Here's the drawing with two shaded views (mm, measured from the low corner). I have some questions. A direction names the side the tool comes from. Coordinates: 2 decimals unless noted, no trailing zeros. Loops run counter-clockwise (first coordinate to the right, second up) from the corner with the lowest first, then second, coordinate; pieces in that order, holes last.
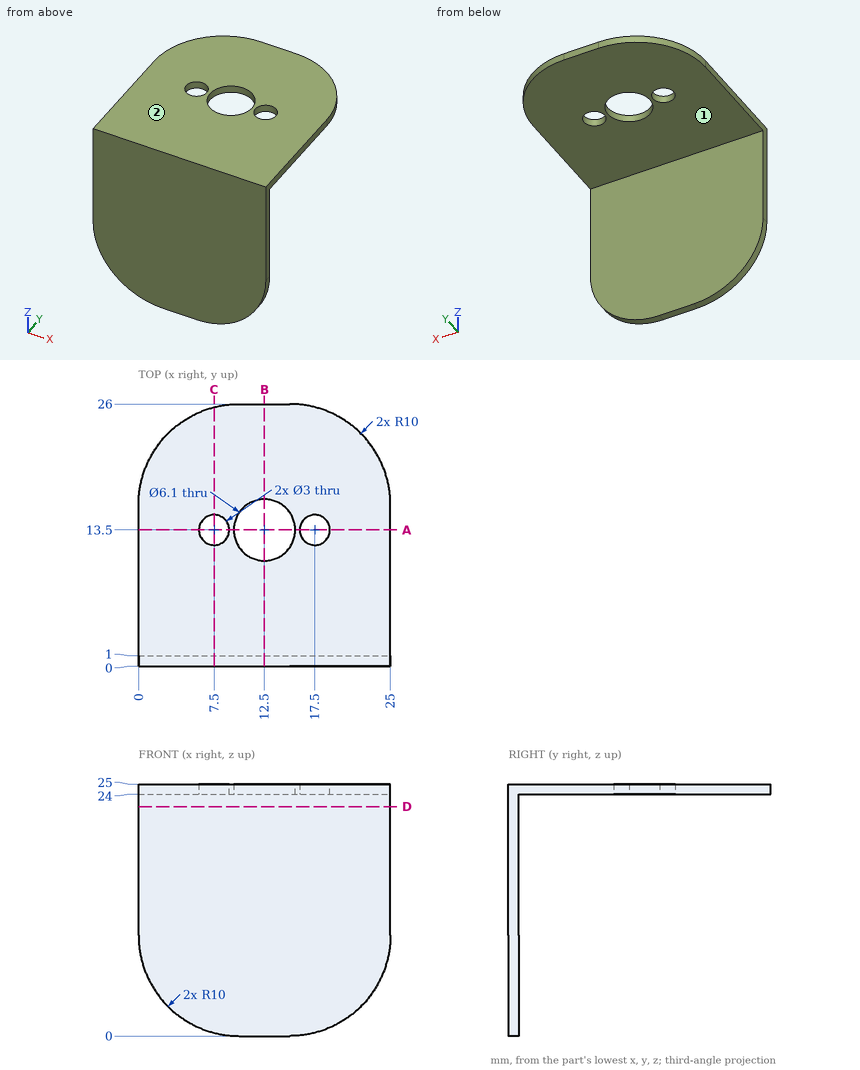
(1) I'm going to push flat-ended pins straight in: pin 1 (2.5 mm diameter, centred on x = 7.5, y = 13.5, fed in from -Z); pin 2 (5 mm diameter, centred on x = 17.5, y = 13.5, fed in from -Z). Where does each tip first touch, or does it pass through?
Check values:
pin 1: passes through
pin 2: stops at z = 24
(2) I want a section at C-C on x = 7.5. Write out the boundary of the cut face in (y, z), then the cut area to 3 significant figures.
Check values:
outline: (0, 0.32) - (1, 0.32) - (1, 24) - (12, 24) - (12, 25) - (0, 25) - close; (15, 24) - (25.68, 24) - (25.68, 25) - (15, 25) - close
area: 46.4 mm2
(3) I want a section at B-B on x = 12.5. Write out the boundary of the cut face in (y, z), then the cut area to 3 significant figures.
Check values:
outline: (0, 0) - (1, 0) - (1, 24) - (10.45, 24) - (10.45, 25) - (0, 25) - close; (16.55, 24) - (26, 24) - (26, 25) - (16.55, 25) - close
area: 43.9 mm2
(4) I want a section at A-A on y = 13.5. Write out the boundary of the cut face in (x, z), then the cut area to 3 significant figures.
Check values:
outline: (0, 24) - (6, 24) - (6, 25) - (0, 25) - close; (9, 24) - (9.45, 24) - (9.45, 25) - (9, 25) - close; (15.55, 24) - (16, 24) - (16, 25) - (15.55, 25) - close; (19, 24) - (25, 24) - (25, 25) - (19, 25) - close
area: 12.9 mm2
(5) I want a section at D-D on z = 22.75. Write out the boundary of the cut face in (x, y), then the cut area to 3 significant figures.
Check values:
outline: (0, 0) - (25, 0) - (25, 1) - (0, 1) - close
area: 25.0 mm2
(6) Which directions (+Z, -Z, +X, -X, +Y, -Y) give clear straight access to the entire face, cutting with the end or side of a thin tool? Please do the marked faces 1 and 2.
Check values:
face 1: -Z, +X, -X, +Y
face 2: +Z, +X, -X, +Y, -Y
(7) If I drill on probe 1 along Z at (x, y) = (2.25, 3.75); probe 2 along Y at (x, z) = (12.5, 24.75); probe 3 along Y at (x, z) = (15, 13.5), over which ranges is the centre line in solid material (lowest first)?
Check values:
probe 1: z = 24 to 25
probe 2: y = 0 to 10.45, 16.55 to 26
probe 3: y = 0 to 1
